from build123d import *

# Parameters (mm, degrees)
CROQUIS1_R                 = 9
CROQUIS1_R_2               = 1.625
SALIENTE_EXTRUIR1_DEPTH    = 8.9
SALIENTE_EXTRUIR2_START    = 20.7
CROQUIS2_R                 = 9
CROQUIS2_R_2               = 7
SALIENTE_EXTRUIR2_DEPTH    = 20.7
CORTAR_EXTRUIR1_DEPTH      = 6.25
CORTAR_EXTRUIR2_DEPTH      = 7.25
CORTAR_EXTRUIR2_DEPTH_BACK = 4.25
CROQUIS4_R                 = 1.625
CROQUIS7_R                 = 11
CROQUIS7_R_2               = 7
SALIENTE_EXTRUIR3_DEPTH    = 1.5
SALIENTE_EXTRUIR4_START    = -1.5
CROQUIS8_R                 = 11
CROQUIS8_R_2               = 9
SALIENTE_EXTRUIR4_DEPTH    = 1.5


with BuildPart() as part:
    # Croquis1 → Saliente-Extruir1 (new body)
    with BuildSketch(Plane.XY):
        with Locations((-4.976335362, -25.8)):
            Circle(CROQUIS1_R)
        with Locations((-4.976335362, -25.8)):
            Circle(CROQUIS1_R_2, mode=Mode.SUBTRACT)
    extrude(amount=-SALIENTE_EXTRUIR1_DEPTH)

    # Croquis2 → Saliente-Extruir2 (add)
    with BuildSketch(Plane.XY.offset(SALIENTE_EXTRUIR2_START)):
        with Locations((-4.976335362, -25.8)):
            Circle(CROQUIS2_R)
        with Locations((-4.976335362, -25.8)):
            Circle(CROQUIS2_R_2, mode=Mode.SUBTRACT)
    extrude(amount=-SALIENTE_EXTRUIR2_DEPTH)

    # Croquis3 → Cortar-Extruir1 (cut)
    with BuildSketch(Plane(origin=(0, 0, -8.9), x_dir=(-1, 0, 0), z_dir=(0, 0, -1))):
        Polygon((8.146335362, -29.3), (8.146335362, -32.3), (1.806335362, -32.3), (1.806335362, -29.3), (4.976335362, -29.3), align=None)
    extrude(amount=-CORTAR_EXTRUIR1_DEPTH, mode=Mode.SUBTRACT)

    # Croquis4 → Cortar-Extruir2 (cut, two sides: drawn at the far end of the back side and taken through both)
    with BuildSketch(Plane.XZ.offset(29.3).offset(-CORTAR_EXTRUIR2_DEPTH_BACK)):
        with Locations(Location((-4.976335362, -5.775, 0), (0, 0, 90))):
            Circle(CROQUIS4_R)
    extrude(amount=CORTAR_EXTRUIR2_DEPTH + CORTAR_EXTRUIR2_DEPTH_BACK, mode=Mode.SUBTRACT)

    # Croquis7 → Saliente-Extruir3 (add)
    with BuildSketch(Plane.XY.offset(20.7)):
        with Locations((-4.976335362, -25.8)):
            Circle(CROQUIS7_R)
        with Locations((-4.976335362, -25.8)):
            Circle(CROQUIS7_R_2, mode=Mode.SUBTRACT)
    extrude(amount=-SALIENTE_EXTRUIR3_DEPTH)

    # Croquis8 → Saliente-Extruir4 (add)
    with BuildSketch(Plane(origin=(0, 0, -8.9), x_dir=(-1, 0, 0), z_dir=(0, 0, -1)).offset(SALIENTE_EXTRUIR4_START)):
        with Locations(Location((4.976335362, -25.8, 0), (0, 0, 180))):
            Circle(CROQUIS8_R)
        with Locations(Location((4.976335362, -25.8, 0), (0, 0, 180))):
            Circle(CROQUIS8_R_2, mode=Mode.SUBTRACT)
    extrude(amount=SALIENTE_EXTRUIR4_DEPTH)


solid = part.part
For this review, take the finished solid that the model builds, in its own axes (mm). A direction names the side the tool comes from. Coordinates: 2 decimals unless noted, no trailing zeros. Loops run counter-clockwise (first coordinate to the right, second up) from the corner with the lowest first, then second, coordinate; pieces in that order, holes last. Notation, with made-up numbers: (-3.75, -19) - (46.25, -19) arc R9 ccw to (46.25, -5) - close; hole circle Ø2 at (23, 68.25). An arc over 180 degrees is marked (long way). Return JSON: item names as keys, results as strings.
Item 1: Take a section at A-A (y = -27). Give the boundary of the cut face in (x, z) (3 decimals), then the cut area to 3 significant figures.
Determined:
{"outline": "(-15.911, -8.9) - (-6.072, -8.9) - (-6.072, -6.975) arc R1.625 cw to (-6.072, -4.575) - (-6.072, 0) - (-11.873, 0) - (-11.873, 20.7) - (-15.911, 20.7) - (-15.911, 19.2) - (-13.896, 19.2) - (-13.896, -7.4) - (-15.911, -7.4) - close; (-3.881, -8.9) - (5.958, -8.9) - (5.958, -7.4) - (3.943, -7.4) - (3.943, 19.2) - (5.958, 19.2) - (5.958, 20.7) - (1.92, 20.7) - (1.92, 0) - (-3.881, 0) - (-3.881, -4.575) arc R1.625 cw to (-3.881, -6.975) - close", "area": "233 mm2"}
Item 2: Insertion check: pin 1 (0.9 mm diameter, centred on x = -4.5, y = -31, fed in from -Z); pin 2 (3.5 mm diameter, centred on y = -31.5, z = -6, fed in from +X); pin 3 (7 mm diameter, centred on x = -5.5, z = -7.5, fed in from +Y); pin 4 (1 mm diameter, centred on x = -9, z = 10, fed in from +Y). Each pin has a flat end and moves straight along its axis. Give the tip position at first contact, or say it passes through.
Determined:
{"pin 1": "stops at z = -2.65", "pin 2": "stops at x = 4.99", "pin 3": "stops at y = -14.8", "pin 4": "stops at y = -17.52"}
Item 3: Take a section at B-B (x = -4.5). State how many separate pieces and enclosed holes the cut face has, then the cut area to 3 significant figures.
Determined:
{"separate pieces": "4", "enclosed holes": "0", "area": "195 mm2"}
Item 4: Mouldability with a two-part tool opening along X and no side actions: class faces 5 (the flat face through (-14, -27.5, -7.4)), 6 (the cylindrical face through (-6.927, -34.586, 6.086)), 7 (the cylindrical face through (-5.464, -33.533, -4.225)) as pulls with the +X half, pulls with the -X half, needs draft (parallel to the pull), parting line crosses it, or undercut.
Determined:
{"face 5": "needs draft", "face 6": "parting line crosses it", "face 7": "undercut"}
Item 5: For line 1 (X direction, y = -25.8, z = -4.75); line 2 (Z direction, x = 2, y = -18.5); line 3 (Y direction, x = -1.25, z = 16.25), list the stretches that pass through material, from the lowest coordinate up.
Determined:
{"line 1": "x = -13.98 to -6.6, -3.35 to 4.02", "line 2": "z = -8.9 to -7.4, 19.2 to 20.7", "line 3": "y = -33.99 to -31.73, -19.87 to -17.61"}
Item 6: For faces 1 (the cylindrical face through (-5, -27.9, -7.4)), 2 (the cylindrical face through (-11.97, -25.49, 10.49)), 3 (the flat face through (-6.4, -32.3, -7.2)), 4 (the flat face through (-3, -35, 19.2)), list the 3-axis set-ups (+Z, -Z, +X, -X, +Y, -Y) from which the entire face can be reached by the end or side of a thin tool; tool diameter is ignored.
Determined:
{"face 1": "-Y", "face 2": "+Z", "face 3": "-Z", "face 4": "none"}
Item 7: Take a section at C-C (z = 4.25). Give the boundary of the cut face in (x, y).
Determined:
{"outline": "circle Ø18 at (-4.98, -25.8); hole circle Ø14 at (-4.98, -25.8)"}
Item 8: Take a section at D-D (x = -1). Give the boundary of the cut face in (y, z), then the cut area to 3 significant figures.
Determined:
{"outline": "(-36.06, -8.9) - (-15.54, -8.9) - (-15.54, -7.4) - (-17.73, -7.4) - (-17.73, 19.2) - (-15.54, 19.2) - (-15.54, 20.7) - (-20.04, 20.7) - (-20.04, 0) - (-31.56, 0) - (-31.56, 20.7) - (-36.06, 20.7) - (-36.06, 19.2) - (-33.87, 19.2) - (-33.87, -7.4) - (-36.06, -7.4) - close", "area": "253 mm2"}
